Input: part model. Units: mm. Frame: model coordinates. A direction names the side the tool comes from. Round coordinates to 2 decimals unless told otherwise and drop trailing zeros. Write each loop counter-clockwise with the first axis right and the second up, starting at its lowest first coordinate (ties: lowest second). Pieces come first, ordered by that corner, then holes. Notation, with made-up numbers: (-24.75, 49) -> (4.25, 49) arc R21 ccw to (4.25, 76) -> close; hole circle Ø3 at (80.5, 4.25). An arc over 180 degrees is marked (long way). Write item = value, one per line.
```python
from build123d import *

# Parameters (mm, degrees)
F1_DEPTH      = 25
F2_W          = 85
F2_H          = 40
F3_DEPTH      = 15
F4_R          = 5
F5_DEPTH      = 15
F5_DEPTH_BACK = 25
F6_R          = 34
F7_DEPTH      = 15
F7_DEPTH_BACK = 15
F8_R          = 23
F9_DEPTH      = 25
F10_R         = 5
F11_DEPTH     = 25


with BuildPart() as f1:
    # F0 (on Top) → F1 (new body)
    with BuildSketch(Plane.XY):
        with BuildLine():
            Line((60, -70), (60, 0))
            ThreePointArc((60, 0), (0, -60), (-60, 0))
            Line((-60, 0), (-60, -70))
            Line((-60, -70), (60, -70))
        make_face()
        with BuildLine():
            ThreePointArc((-60, 0), (0, -60), (60, 0))
            Line((60, 0), (-60, 0))
        make_face()
        with BuildLine():
            Line((-60, 0), (60, 0))
            ThreePointArc((60, 0), (0, 60), (-60, 0))
        make_face()
    extrude(amount=-F1_DEPTH)

    # F2 (on Top) → F3 (join)
    with BuildSketch(Plane.XY):
        with Locations((0, -50)):
            Rectangle(F2_W, F2_H)
    extrude(amount=F3_DEPTH)

    # F4 (on Top) → F5 (cut, two sides)
    with BuildSketch(Plane.XY) as f5_sk:
        with Locations((0, -50)):
            Circle(F4_R)
    extrude(amount=F5_DEPTH, mode=Mode.SUBTRACT)
    extrude(f5_sk.sketch, amount=-F5_DEPTH_BACK, mode=Mode.SUBTRACT)

    # F6 (on Top) → F7 (cut, two sides)
    with BuildSketch(Plane.XY) as f7_sk:
        Circle(F6_R)
    extrude(amount=-F7_DEPTH, mode=Mode.SUBTRACT)
    extrude(f7_sk.sketch, amount=F7_DEPTH_BACK, mode=Mode.SUBTRACT)

    # F8 (on Top) → F9 (cut)
    with BuildSketch(Plane.XY):
        Circle(F8_R)
    extrude(amount=-F9_DEPTH, mode=Mode.SUBTRACT)

    # F10 (on Top) → F11 (cut)
    with BuildSketch(Plane.XY):
        with Locations((-50, 0)):
            Circle(F10_R)
        with Locations((0, 50)):
            Circle(F10_R)
        with Locations((50, 0)):
            Circle(F10_R)
    extrude(amount=-F11_DEPTH, mode=Mode.SUBTRACT)


solid = f1.part
```
1) Draft query along Y for faces 5 (the face through (-42.5, -50, 7)), 6 (the face through (-29, -30, 7)), 7 (the face through (-0.651, 54.957, -12.325)). Return one class per face: +Y half, -Y half, draft (parallel to the pull), parting line (faces both ways), or undercut.
Solutions:
face_5 = draft
face_6 = +Y half
face_7 = undercut
2) First-contact query: P1, Ø12, axis at x = -12, y = -15.5, coming from the +Z side; P2, Ø11.5, axis at x = -50, y = 0, coming from the +Z side; P3, Ø12, axis at y = -55, z = 7, coming from the -X side. Flat tips, straight axial feed; report the tip coordinate or a pass-through.
Solutions:
P1 = -15
P2 = 0
P3 = -42.5
3) Line query: L1, parallel to Y at x = 0, z = -6.75; L2, parallel to Y at x = 0, z = -18; L3, parallel to Z at x = 43, y = -9.5. Output: solid intervals per line, ascending. Write a range as from..to.
Solutions:
L1 = -70..-55, -45..-34, 34..45, 55..60
L2 = -70..-55, -45..-23, 23..45, 55..60
L3 = -25..0
4) Cut plane B-B (x = 0). Return the cut outline in (y, z).
Solutions:
outline = (-70, -25) -> (-55, -25) -> (-55, 15) -> (-70, 15) -> close; (-45, -25) -> (-23, -25) -> (-23, -15) -> (-34, -15) -> (-34, 15) -> (-45, 15) -> close; (23, -25) -> (45, -25) -> (45, 0) -> (34, 0) -> (34, -15) -> (23, -15) -> close; (55, -25) -> (60, -25) -> (60, 0) -> (55, 0) -> close
5) Cut plane C-C (z = -8.5). Return the cut outline in (x, y), and give its area (3 significant figures).
Solutions:
outline = (-60, -70) -> (60, -70) -> (60, 0) arc R60 ccw to (-60, 0) -> close; hole circle Ø10 at (-50, 0); hole circle Ø68 at (0, 0); hole circle Ø10 at (0, -50); hole circle Ø10 at (0, 50); hole circle Ø10 at (50, 0)
area = 10,100 mm^2
6) Cut plane A-A (y = -50). Return the cut outline in (x, z).
Solutions:
outline = (-60, -25) -> (-5, -25) -> (-5, 15) -> (-42.5, 15) -> (-42.5, 0) -> (-60, 0) -> close; (5, -25) -> (60, -25) -> (60, 0) -> (42.5, 0) -> (42.5, 15) -> (5, 15) -> close
7) Access query for faces 1 (the face through (42.5, -50, 7)), 2 (the face through (60, -35, -12)), 3 (the face through (29, -30, 7)), 4 (the face through (-7.37, -33.19, -6.46)). Directions: +Z, -Z, +X, -X, +Y, -Y. A direction counts if a zero-diameter tool reaches every point of the face in a straight line with its end or side. Return the directions, or none.
Solutions:
face_1 = +Z, +X, +Y, -Y
face_2 = +Z, -Z, +X, +Y, -Y
face_3 = +Z, +X, -X, +Y
face_4 = +Z
8) Cut plane D-D (z = 9.5). Return the cut outline in (x, y), and give its area (3 significant figures).
Solutions:
outline = (-42.5, -70) -> (42.5, -70) -> (42.5, -30) -> (16, -30) arc R34 cw to (-16, -30) -> (-42.5, -30) -> close; hole circle Ø10 at (0, -50)
area = 3,240 mm^2
